Answer from the drawing. Dimensions are ordinates in mm from the lowest x, y and z of the part. A direction names the side the tool comes from. Coordinates: 2 decimals unless noted, no trailing zeros. Loops run counter-clockwise (first coordinate to the right, second up) from the corner with the lowest first, then second, coordinate; pieces in that order, holes last. Notation, with made-up numbers: (4.25, -14) - (9.25, -14) arc R26 cw to (9.25, 17) - close; hole circle Ø11 at (-22, 66.25). An arc over 180 degrees is marked (long way). Use one line per item in the form item = value. Start each with the question number.
1) Consider line 1 (Z direction, x = 1.1, y = 15.25); line 2 (Y direction, x = 1.35, z = 6.75); line 3 (Y direction, x = 2, z = 3.5) (1 decimal). Determine where each line is inside the solid, lowest interval first.
2) A cutting plane is placed at B-B (x = 3). Give the vertices of the cut face in (y, z).
3) A cutting plane is placed at C-C (y = 13.75). Give the vertices of the cut face in (x, z) (1 decimal), and give its area (3 significant figures).
4) Which of the six approach directions +Z, -Z, +X, -X, +Y, -Y give full straight-line access (tool end or side, diameter ignored) to the marked faces 1, 2, 3, 4 and 5?
5) Each of these flat-tipped pins is pushed along its axis until it touches: P1, Ø1.1, axis at y = 14.5, z = 9, coming from the -X side; P2, Ø1, axis at x = 2.5, y = 13, coming from the -Z side; P3, Ø1.7, axis at x = 2, y = 13.5, coming from the +Z side; P4, Ø1.6, axis at y = 14.5, z = 8.5, coming from the +X side. Where does it stop, or does it pass through?
6) A cutting plane is placed at A-A (z = 3.5). Give the vertices of the cut face in (x, y).
7) A cutting plane is placed at D-D (z = 8.5). Give the vertices of the cut face in (x, y).
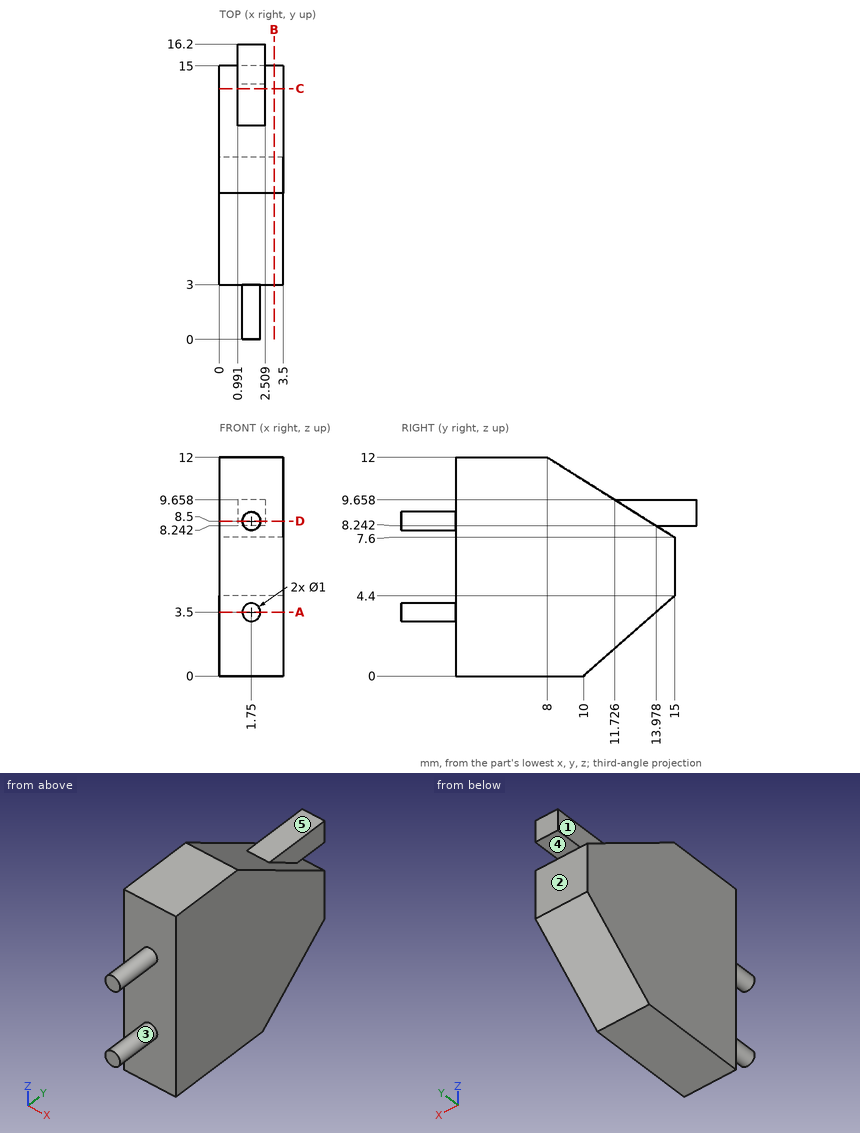
Found:
q1.line_1 = 8.24 to 9.66
q1.line_2 = 3 to 15
q1.line_3 = 0 to 14
q2.outline = (3, 0) - (10, 0) - (15, 4.4) - (15, 7.6) - (8, 12) - (3, 12) - close
q3.outline = (0, 3.3) - (3.5, 3.3) - (3.5, 8.4) - (2.5, 8.4) - (2.5, 9.7) - (1, 9.7) - (1, 8.4) - (0, 8.4) - close
q3.area = 19.7 mm^2
q4.face_1 = +Z, -X, +Y
q4.face_2 = -Z, +X, -X, +Y
q4.face_3 = -Y
q4.face_4 = +X, -X, +Y
q4.face_5 = +Z, +X, -X, +Y
q5.P1 = 0.99
q5.P2 = 2.2
q5.P3 = 9.66
q5.P4 = 3.5
q6.outline = (0, 3) - (1.25, 3) - (1.25, 0) - (2.25, 0) - (2.25, 3) - (3.5, 3) - (3.5, 13.98) - (0, 13.98) - close
q7.outline = (0, 3) - (1.25, 3) - (1.25, 0) - (2.25, 0) - (2.25, 3) - (3.5, 3) - (3.5, 13.57) - (2.51, 13.57) - (2.51, 16.2) - (0.99, 16.2) - (0.99, 13.57) - (0, 13.57) - close
